```python
from build123d import *

# Parameters (mm, degrees)
BOSS_EXTRUDE3_DEPTH      = 6.35
BOSS_EXTRUDE3_DEPTH_BACK = 6.35
SKETCH3_R                = 28.575
BOSS_EXTRUDE4_DEPTH      = 19.05
BOSS_EXTRUDE4_DEPTH_BACK = 19.05
SKETCH4_R                = 6.35
CUT_EXTRUDE1_DEPTH       = 26.4
SKETCH5_R                = 14.2875
CUT_EXTRUDE2_DEPTH       = 39.1
SKETCH6_W                = 17.4752
SKETCH6_H                = 6.35
CUT_EXTRUDE3_DEPTH       = 39.1


with BuildPart() as part:
    # Sketch1 → Boss-Extrude3 (new body, two sides)
    with BuildSketch(Plane.XY) as boss_extrude3_sk:
        with BuildLine():
            Line((4.396153846, -28.234809303), (84.992307692, -15.686005168))
            ThreePointArc((84.992307692, -15.686005168), (98.425, 0), (84.992307692, 15.686005168))
            Line((84.992307692, 15.686005168), (4.396153846, 28.234809303))
            ThreePointArc((4.396153846, 28.234809303), (28.575, 0), (4.396153846, -28.234809303))
        make_face()
    extrude(amount=BOSS_EXTRUDE3_DEPTH)
    extrude(boss_extrude3_sk.sketch, amount=-BOSS_EXTRUDE3_DEPTH_BACK)

    # Sketch3 → Boss-Extrude4 (add, two sides)
    with BuildSketch(Plane.XY) as boss_extrude4_sk:
        Circle(SKETCH3_R)
    extrude(amount=BOSS_EXTRUDE4_DEPTH)
    extrude(boss_extrude4_sk.sketch, amount=-BOSS_EXTRUDE4_DEPTH_BACK)

    # Sketch4 → Cut-Extrude1 (cut, through all)
    with BuildSketch(Plane.XY.offset(6.35)):
        with Locations((82.55, 0)):
            Circle(SKETCH4_R)
    extrude(amount=-CUT_EXTRUDE1_DEPTH, mode=Mode.SUBTRACT)

    # Sketch5 → Cut-Extrude2 (cut, through all)
    with BuildSketch(Plane.XY.offset(19.05)):
        Circle(SKETCH5_R)
    extrude(amount=-CUT_EXTRUDE2_DEPTH, mode=Mode.SUBTRACT)

    # Sketch6 → Cut-Extrude3 (cut, through all)
    with BuildSketch(Plane.XY.offset(19.05)):
        with Locations((8.7376, 0)):
            Rectangle(SKETCH6_W, SKETCH6_H)
    extrude(amount=-CUT_EXTRUDE3_DEPTH, mode=Mode.SUBTRACT)


solid = part.part
```
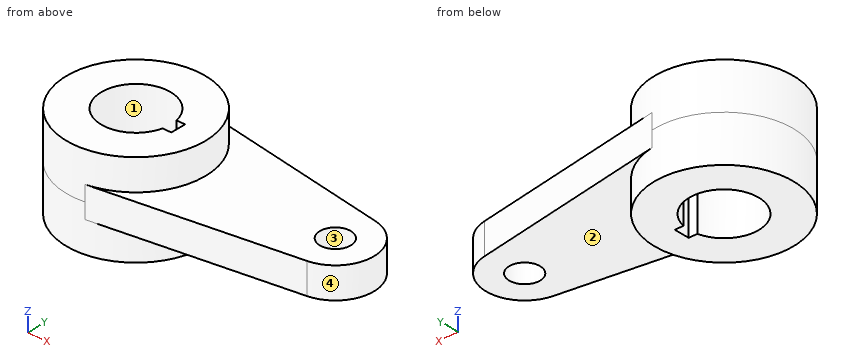
The model under review builds one solid part; all positions refer to its coordinate system, in mm. Face numbers are marked on the shaded views. Give positions to 0.01 mm unless a question says otherwise; leave off trailing zeros. Order: outer loops, then holes, each group sorted by start corner. A loop starts at its lowest first (then second) coordinate and runs counter-clockwise, first axis right, second up. Notation, with made-up numbers: (-34.5, 47) - (-29.5, 47) arc R13 cw to (-29.5, 62) - close; hole circle Ø6 at (16.5, 64.25). An arc over 180 degrees is marked (long way). Use CSV: the item, a comma, the result in double quotes. Start each with the question number.
Q1. To check wall thickness, follow line 1 along Y through (x, z) = (0, 3.5) (1 decimal); line 2 along X through (y, z) = (0.5, -6.5); line 3 along Z through (x, y) = (34, -2.5). State the ranges of each line that lie inside material, in increasing order. Write a range as [from, to].
Q2. Clearance check with flat-ended pins moving along their axes: pin 1 Ø5 at (x, z) = (9, 8) entering from +Y; pin 2 Ø1.5 at (y, z) = (-22.5, 6.5) entering from -X; pin 3 Ø10 at (x, y) = (50.5, 16.5) entering from +Z. State where each tip first meets the part, or that it passes through.
Q3. We need section B-B, the plane y = -11.5. Write out the cut boundary in (x, z), and give its area (3 significant figures).
Q4. The part is to be moulded in two halves that separate along X. For the marked faces 1, 2, 3 and 4, say which applies: +X half, -X half, draft (parallel to the pull), parting line (faces both ways), or undercut.
Q5. We need section C-C, the plane z = -5. State how many separate pieces and enclosed holes the cut face has, and give its area (3 significant figures).
Outcome:
1,line 1,"y = [-28.6, -14.3], [14.3, 28.6]"
1,line 2,"x = [-28.57, -14.28], [17.48, 28.57]"
1,line 3,"z = [-6.35, 6.35]"
2,pin 1,"stops at y = 27.83"
2,pin 2,"stops at x = -18.53"
2,pin 3,"stops at z = 6.35"
3,outline,"(-26.16, -19.05) - (-8.48, -19.05) - (-8.48, 19.05) - (-26.16, 19.05) - close; (8.48, -19.05) - (26.16, -19.05) - (26.16, -6.35) - (93.49, -6.35) - (93.49, 6.35) - (26.16, 6.35) - (26.16, 19.05) - (8.48, 19.05) - close"
3,area,"2,200 mm^2"
4,face 1,"undercut"
4,face 2,"draft"
4,face 3,"undercut"
4,face 4,"+X half"
5,separate pieces,"1"
5,enclosed holes,"2"
5,area,"4,600 mm^2"
